Here's how the part is built. I have some questions about the finished solid (model axes, mm). A direction names the side the tool comes from. Round coordinates to 2 decimals unless told otherwise and drop trailing zeros. Loops run counter-clockwise (first coordinate to the right, second up) from the corner with the lowest first, then second, coordinate; pieces in that order, holes last. Notation, with made-up numbers: (38, -9) - (78, -9) arc R27 cw to (78, 20) - close; hole circle Ø1 at (-7.5, 33.25). An arc over 180 degrees is marked (long way). Return JSON: item names as keys, results as strings. Group by question number.
```python
from build123d import *

# Parameters (mm, degrees)
SKETCH_R              = 82.55
PAD_DEPTH             = 12.7
SKETCH001_R           = 10
POCKET_DEPTH          = 12.701
SKETCH002_R           = 30.25
SKETCH002_R_2         = 26
POCKET001_DEPTH       = 7
SKETCH003_R           = 3.175
POCKET002_DEPTH       = 480.364597
POLARPATTERN_COUNT    = 6
POCKET003_DEPTH       = 5
POLARPATTERN001_COUNT = 6


with BuildPart() as part:
    # Sketch → Pad (new body)
    with BuildSketch(Plane.XY):
        Circle(SKETCH_R)
    extrude(amount=-PAD_DEPTH)

    # Sketch001 (on Face2 of Pad) → Pocket (cut, through all)
    with BuildSketch(Plane.XY):
        Circle(SKETCH001_R)
    extrude(amount=-POCKET_DEPTH, mode=Mode.SUBTRACT)

    # Sketch002 (on Face2 of Pocket) → Pocket001 (cut)
    with BuildSketch(Plane.XY):
        Circle(SKETCH002_R)
        Circle(SKETCH002_R_2, mode=Mode.SUBTRACT)
    extrude(amount=-POCKET001_DEPTH, mode=Mode.SUBTRACT)

    # Sketch003 (on Face2 of Pocket001) → Pocket002 (cut, through all)
    with BuildSketch(Plane.XY):
        with Locations((0, -70)):
            Circle(SKETCH003_R)
    pocket002 = extrude(amount=-POCKET002_DEPTH, mode=Mode.SUBTRACT)

    # PolarPattern: Pocket002 ×6 about axis
    polarpattern_axis = Axis((0, 0, 0), (0, 0, 1))
    for i in range(1, POLARPATTERN_COUNT):
        add(pocket002.rotate(polarpattern_axis, i * 360 / POLARPATTERN_COUNT), mode=Mode.SUBTRACT)

    # Sketch004 (on Face2 of PolarPattern) → Pocket003 (cut)
    with BuildSketch(Plane.XY):
        with BuildLine():
            ThreePointArc((-70, 5.5), (-75.5, 0), (-70, -5.5))
            Line((-70, -5.5), (-45, -5.5))
            ThreePointArc((-45, -5.5), (-39.5, 0), (-45, 5.5))
            Line((-70, 5.5), (-45, 5.5))
        make_face()
    pocket003 = extrude(amount=-POCKET003_DEPTH, mode=Mode.SUBTRACT)

    # PolarPattern001: Pocket003 ×6 about axis
    polarpattern001_axis = Axis((0, 0, 0), (0, 0, 1))
    for i in range(1, POLARPATTERN001_COUNT):
        add(pocket003.rotate(polarpattern001_axis, i * 360 / POLARPATTERN001_COUNT), mode=Mode.SUBTRACT)


solid = part.part
```
Q1. If we mould it in two halves opening along X, with no side actions, what happens to faces 1 (the flat face through (-1, -36, 0)), 2 (the flat face through (-33.6, 47.2, -2.5))? For each: +X half, -X half, draft (parallel to the pull), parting line (faces both ways), or undercut.
Q2. Imagine slicing it at C-C, the plane z = -2.5. Give the number of separate pieces and of enclosed holes in the cut face, and give its area (3 significant figures).
Q3. Imagine slicing it at D-D, the plane y = -60.5. List the corners of the cut face in (x, z) for me.
Q4. Imagine slicing it at A-A, the plane x = 0. List the corners of the cut face in (y, z) for me (3 decimals).
Q5. Imagine slicing it at B-B, the plane y = 70. List the corners of the cut face in (x, z) for me (3 decimals).
Q6. Please list where these lines run through material, in increasing order: line 1 (Y direction, x = -38, z = -4.75); line 2 (Y direction, x = 62, z = -1.25); line 3 (Y direction, x = 61.5, z = -4).
Q7. Will these pins go through, and if not, where does the flat tip stop? pin 1 Ø5.5 at (x, z) = (-58, -2.5) entering from -Y; pin 2 Ø1.5 at (y, z) = (-15.5, -6) entering from +X; pin 3 Ø4 at (x, z) = (12.5, -2) entering from +Y.
Q8. For faces 3 (the flat face through (-29, -50, -5)), 4 (the cylindrical face through (59.16, -32.18, -6.26)), which set-ups out of +Z, -Z, +X, -X, +Y, -Y let a thin tool reach every point of the face, with its end or its side?
Output values:
{
 "1": {"face 1": "draft", "face 2": "undercut"},
 "2": {"separate pieces": "2", "enclosed holes": "14", "area": "17,900 mm^2"},
 "3": {"outline": "(-56.16, -12.7) - (56.16, -12.7) - (56.16, 0) - (40.5, 0) - (40.5, -5) - (28.58, -5) - (28.58, 0) - (-28.58, 0) - (-28.58, -5) - (-40.5, -5) - (-40.5, 0) - (-56.16, 0) - close"},
 "4": {"outline": "(-82.55, -12.7) - (-73.175, -12.7) - (-73.175, 0) - (-82.55, 0) - close; (-66.825, -12.7) - (-10, -12.7) - (-10, 0) - (-26, 0) - (-26, -7) - (-30.25, -7) - (-30.25, 0) - (-66.825, 0) - close; (10, -12.7) - (66.825, -12.7) - (66.825, 0) - (30.25, 0) - (30.25, -7) - (26, -7) - (26, 0) - (10, 0) - close; (73.175, -12.7) - (82.55, -12.7) - (82.55, 0) - (73.175, 0) - close"},
 "5": {"outline": "(-43.755, -12.7) - (-3.175, -12.7) - (-3.175, 0) - (-43.755, 0) - close; (3.175, -12.7) - (43.755, -12.7) - (43.755, 0) - (3.175, 0) - close"},
 "6": {"line 1": "y = -73.28 to -65.23, -54.82 to 54.82, 65.23 to 73.28", "line 2": "y = -54.5 to -37.86, -32.14 to -5.5, 5.5 to 32.14, 37.86 to 54.5", "line 3": "y = -55.07 to -38.05, -31.95 to -5.5, 5.5 to 31.95, 38.05 to 55.07"},
 "7": {"pin 1": "stops at y = -61.33", "pin 2": "stops at x = 81.22", "pin 3": "stops at y = 81.88"},
 "8": {"face 3": "+Z", "face 4": "+Z, -Z"}
}
